```python
from build123d import *

# Parameters (mm, degrees)
CAP_SKETCH_W            = 20
CAP_SKETCH_H            = 40
EXTRUDE_THICKNESS_DEPTH = 2
CORNER_FILLETS_R        = 1
TOP_EDGE_FILLET_R       = 1


with BuildPart() as part:
    # Cap Sketch → Extrude Thickness (new body)
    with BuildSketch(Plane.XY):
        Rectangle(CAP_SKETCH_W, CAP_SKETCH_H)
    extrude(amount=EXTRUDE_THICKNESS_DEPTH)

    # Corner Fillets
    corner_fillets_edges = [part.edges().sort_by_distance(p)[0] for p in [
        (10, -20, 1),
        (-10, -20, 1),
        (-10, 20, 1),
        (10, 20, 1),
    ]]
    fillet(corner_fillets_edges, radius=CORNER_FILLETS_R)

    # Top Edge Fillet
    top_edge_fillet_edges = [part.edges().sort_by_distance(p)[0] for p in [
        (0, -20, 2),
        (-10, 0, 2),
        (10, 0, 2),
        (0, 20, 2),
        (9.707106781, -19.707106781, 2),
        (9.707106781, 19.707106781, 2),
        (-9.707106781, 19.707106781, 2),
        (-9.707106781, -19.707106781, 2),
    ]]
    fillet(top_edge_fillet_edges, radius=TOP_EDGE_FILLET_R)


solid = part.part
```
Geometry check sheet. Reference: the model listing, model coordinates, mm. Coordinates: 2 decimals unless noted, no trailing zeros. Order: outer loops, then holes, each group sorted by start corner. A loop starts at its lowest first (then second) coordinate and runs counter-clockwise, first axis right, second up. Notation, with made-up numbers: M 0.25,-28 L 10.25,-28 A27 ccw 10.25,6 Z; hole C -3.5,89.25 d6. An arc over 180 degrees is marked long. Answer as a JSON object with one key per item and string values.
Q1. Depth check by flat-ended pin: pin 1 Ø12 at (x, y) = (-1.5, 12) entering from -Z. Enter the tip coordinate at first touch or a pass-through.
Results are:
{"pin 1": "stops at z = 0"}
Q2. Scan lines: line 1 (Y direction, x = -1.25, z = 1.15); line 2 (X direction, y = -13, z = 1.6); line 3 (X direction, y = 8, z = 1.7). Record each from-to range of solid material in increasing order.
Results are:
{"line 1": "y = -19.99 to 19.99", "line 2": "x = -9.8 to 9.8", "line 3": "x = -9.71 to 9.71"}
Q3. Cross-section at A-A on z = 1.7. Record the cut outline in (x, y).
Results are:
{"outline": "M -9.71,-19 A0.71 ccw -9,-19.71 L 9,-19.71 A0.71 ccw 9.71,-19 L 9.71,19 A0.71 ccw 9,19.71 L -9,19.71 A0.71 ccw -9.71,19 Z"}
